Geometry: final body of the model. Coordinates: model frame, mm. A direction names the side the tool comes from. Round coordinates to 2 decimals unless told otherwise and drop trailing zeros. Write each loop counter-clockwise with the first axis right and the second up, starting at its lowest first coordinate (ties: lowest second). Pieces come first, ordered by that corner, then holes. Notation, with made-up numbers: M 80.25,31.25 L 93.25,31.25 A5 cw 93.25,37.25 Z; hole C -26,70 d7. An arc over 180 degrees is marked long. Answer as CSV lines item,"result". Start each with the question number.
Q1. Ray query, probe 1 along Y at (x, z) = (15, 1.25); probe 2 along X at (y, z) = (-3.5, 13); probe 3 along Y at (x, z) = (-20, 6.25) (3 decimals). Return the intervals inside material, ascending.
Q2. Section query A-A on z = 1.5. Output: boundary loops of the cut face in (x, y) (3 decimals).
Q3. First-contact query: pin 1 (5 mm diameter, centred on x = 20, y = 30, fed in from -Z); pin 2 (6.5 mm diameter, centred on x = -46, y = 1, fed in from +Z); pin 3 (4 mm diameter, centred on x = 44.5, y = 0, fed in from +Z); pin 4 (5 mm diameter, centred on x = 38.5, z = 6.5, fed in from -Y). Flat tips, straight axial feed; report the tip coordinate or a pass-through.
Q4. Section query C-C on z = 6.25. Output: boundary loops of the cut face in (x, y) (3 decimals), and give its area (3 significant figures).
Q5. Section query B-B on y = 11. Output: boundary loops of the cut face in (x, z), and give its area (3 significant figures).
Q6. Section query D-D on y = 28.5. Output: boundary loops of the cut face in (x, z), and give its area (3 significant figures).
Q7. Mould query, pull axis Y, two halves, no side actions, for faces 1 (the cylindrical face through (-47.77, 5.46, 10.11)), 2 (the cylindrical face through (41.82, -2.43, 12.6)), 3 (the cylindrical face through (-50.26, -6.03, 9.86)), 4 (the cylindrical face through (21.688, 14.265, 9.86)). Classes: pulls with the +Y half, pulls with the -Y half, needs draft (parallel to the pull), parting line crosses it, or undercut.
Q8. Reachability of faces 5 (the flat face through (-1, 20, 20)), 6 (the cylindrical face through (-43.154, -3.549, 12.605)), 7 (the flat face through (0, 15, 10)) from +Z, -Z, +X, -X, +Y, -Y: full face, straight path, thin tool, end or side. Return the list, or none.
```python
from build123d import *

# Parameters (mm, degrees)
BOSS_EXTRUDE1_DEPTH = 20
SKETCH2_R           = 4
CUT_EXTRUDE1_DEPTH  = 15
SKETCH6_R           = 2.425
CUT_EXTRUDE5_DEPTH  = 6
CUT_EXTRUDE6_REACH  = 70.213
SKETCH7_R           = 3.175


with BuildPart() as part:
    # Sketch1 → Boss-Extrude1 (new body)
    with BuildSketch(Plane.XY):
        with BuildLine():
            Line((-26.145770237, 35.121475197), (-51.145770237, 5.121475197))
            ThreePointArc((-51.145770237, 5.121475197), (-50.121475197, -6.145770237), (-38.854229763, -5.121475197))
            Line((-38.854229763, -5.121475197), (-24.485104434, 12.121475197))
            ThreePointArc((-24.485104434, 12.121475197), (-21.732577368, 14.24471537), (-18.339334198, 15))
            Line((-18.339334198, 15), (18.339334198, 15))
            ThreePointArc((18.339334198, 15), (21.732577368, 14.24471537), (24.485104434, 12.121475197))
            Line((24.485104434, 12.121475197), (38.854229763, -5.121475197))
            ThreePointArc((38.854229763, -5.121475197), (50.121475197, -6.145770237), (51.145770237, 5.121475197))
            Line((51.145770237, 5.121475197), (26.145770237, 35.121475197))
            ThreePointArc((26.145770237, 35.121475197), (23.39324317, 37.24471537), (20, 38))
            Line((20, 38), (-20, 38))
            ThreePointArc((-20, 38), (-23.39324317, 37.24471537), (-26.145770237, 35.121475197))
        make_face()
    extrude(amount=BOSS_EXTRUDE1_DEPTH)

    # Sketch2 → Cut-Extrude1 (cut)
    with BuildSketch(Plane.XY.offset(20)):
        with Locations((-45, 0)):
            Circle(SKETCH2_R)
        with Locations((44.995948223, 0)):
            Circle(SKETCH2_R)
    extrude(amount=-CUT_EXTRUDE1_DEPTH, mode=Mode.SUBTRACT)

    # Sketch6 → Cut-Extrude5 (cut)
    with BuildSketch(Plane(origin=(-32.703147286, 27.252622738, 0), x_dir=(0, 0, 1), z_dir=(-0.7682212795973757, 0.6401843996644799, 0))):
        with Locations(Location((10, -28.808297985, 0), (0, 0, 270))):
            Circle(SKETCH6_R)
    cut_extrude5 = extrude(amount=-CUT_EXTRUDE5_DEPTH, mode=Mode.SUBTRACT)

    # Mirror2: Cut-Extrude5 across plane
    add(cut_extrude5.mirror(Plane(origin=(0, 0, 0), x_dir=(0, 0, 1), z_dir=(1, 0, 0))), mode=Mode.SUBTRACT)

    # Sketch7 → Cut-Extrude6 (cut, up to next)
    with BuildSketch(Plane.XY.offset(20), mode=Mode.PRIVATE) as cut_extrude6_sk1:
        with Locations((-20, 30)):
            Circle(SKETCH7_R)
    cut_extrude6_tool1 = extrude(cut_extrude6_sk1.sketch, amount=-CUT_EXTRUDE6_REACH, mode=Mode.PRIVATE) & part.part
    # Sketch7 → Cut-Extrude6 (cut, up to next)
    with BuildSketch(Plane.XY.offset(20), mode=Mode.PRIVATE) as cut_extrude6_sk2:
        with Locations((20, 30)):
            Circle(SKETCH7_R)
    cut_extrude6_tool2 = extrude(cut_extrude6_sk2.sketch, amount=-CUT_EXTRUDE6_REACH, mode=Mode.PRIVATE) & part.part
    add(cut_extrude6_tool1.solids().sort_by_distance((-20, 30, 20))[0], mode=Mode.SUBTRACT)
    add(cut_extrude6_tool2.solids().sort_by_distance((20, 30, 20))[0], mode=Mode.SUBTRACT)


solid = part.part
```
Entries:
1,probe 1,"y = 15 to 38"
1,probe 2,"x = -52.19 to -46.94, -43.06 to -37.5, 37.5 to 43.06, 46.93 to 52.19"
1,probe 3,"y = 14.826 to 26.825, 33.175 to 38"
2,outline,"M -51.146,5.121 A8 ccw -38.854,-5.121 L -24.485,12.121 A8 cw -18.339,15 L 18.339,15 A8 cw 24.485,12.121 L 38.854,-5.121 A8 ccw 51.146,5.121 L 26.146,35.121 A8 ccw 20,38 L -20,38 A8 ccw -26.146,35.121 Z; hole C -20,30 d6.35; hole C 20,30 d6.35"
3,pin 1,"passes through"
3,pin 2,"stops at z = 20"
3,pin 3,"stops at z = 5"
3,pin 4,"stops at y = -6.93"
4,outline,"M -51.146,5.121 A8 ccw -38.854,-5.121 L -24.485,12.121 A8 cw -18.339,15 L 18.339,15 A8 cw 24.485,12.121 L 38.854,-5.121 A8 ccw 51.146,5.121 L 26.146,35.121 A8 ccw 20,38 L -20,38 A8 ccw -26.146,35.121 Z; hole C -45,0 d8; hole C -20,30 d6.35; hole C 20,30 d6.35; hole C 44.996,0 d8"
4,area,"2,200 mm^2"
5,outline,"M -46.25,0 L -25.42,0 L -25.42,20 L -46.25,20 Z; M 25.42,0 L 46.25,0 L 46.25,20 L 25.42,20 Z"
5,area,"833 mm^2"
6,outline,"M -31.66,0 L -22.8,0 L -22.8,20 L -31.66,20 Z; M -17.2,0 L 17.2,0 L 17.2,20 L -17.2,20 Z; M 22.8,0 L 31.66,0 L 31.66,20 L 22.8,20 Z"
6,area,"1,040 mm^2"
7,face 1,"undercut"
7,face 2,"undercut"
7,face 3,"parting line crosses it"
7,face 4,"pulls with the -Y half"
8,face 5,"+Z, +X, -X, +Y, -Y"
8,face 6,"+Z"
8,face 7,"+Z, -Z, -Y"
